CAD build for the part. Positions are in the model's coordinates, mm. Give positions to 0.01 mm unless a question says otherwise; leave off trailing zeros. Write each loop counter-clockwise with the first axis right and the second up, starting at its lowest first coordinate (ties: lowest second). Pieces come first, ordered by that corner, then holes. Notation, with made-up numbers: (60, -35) - (87, -35) arc R22 ccw to (87, -26) - close; hole circle Ø3 at (71, -11.5). An arc over 180 degrees is marked (long way). Answer as a JSON object with one key per item and string values.
from build123d import *

# Parameters (mm, degrees)
F0_R     = 10
F0_R_2   = 5
F1_DEPTH = 5
F3_DEPTH = 15
F4_R     = 5
F5_DEPTH = 24.90763


with BuildPart() as f1:
    # F0 (on Front) → F1 (new body)
    with BuildSketch(Plane.XZ):
        Circle(F0_R)
        Circle(F0_R_2, mode=Mode.SUBTRACT)
    extrude(amount=F1_DEPTH)

    # F2 (on Front) → F3 (join)
    with BuildSketch(Plane.XZ):
        with BuildLine():
            ThreePointArc((0, -10), (7.071068, -7.071068), (10, 0))
            ThreePointArc((10, 0), (7.071068, 7.071068), (0, 10))
            ThreePointArc((0, 10), (-10, 0), (0, -10))
        make_face()
        with BuildLine():
            ThreePointArc((0, 10), (7.071068, 7.071068), (10, 0))
            ThreePointArc((10, 0), (7.071068, -7.071068), (0, -10))
            Line((0, -10), (15, -10))
            Line((15, -10), (23.552744, -5))
            Line((23.552744, -5), (23.552744, 5))
            Line((23.552744, 5), (15, 10))
            Line((15, 10), (0, 10))
        make_face()
    extrude(amount=-F3_DEPTH)

    # F4 (on Front) → F5 (cut, symmetric)
    with BuildSketch(Plane.XZ):
        Circle(F4_R)
    extrude(amount=F5_DEPTH, both=True, mode=Mode.SUBTRACT)


solid = f1.part
(1) Saw through at B-B, the plane x = -4. Give the cut face in (y, z), and give its area (3 significant figures).
Answer key:
{"outline": "(-5, -9.17) - (15, -9.17) - (15, -3) - (-5, -3) - close; (-5, 3) - (15, 3) - (15, 9.17) - (-5, 9.17) - close", "area": "247 mm²"}
(2) Saw through at C-C, the plane y = 10.5. Give the cut face in (x, z).
Answer key:
{"outline": "(0, -10) - (15, -10) - (23.55, -5) - (23.55, 5) - (15, 10) - (0, 10) arc R10 ccw to start; hole circle Ø10 at (0, 0)"}
(3) Probe L1, parallel to Z at x = 0, y = -3.2; L2, parallel to Y at x = 16.5, z = 8; L3, parallel to X at y = 2.5, z = 1. List the from-to ranges inside material, lowest first. Write a range as [from, to].
Answer key:
{"L1": "z = [-10, -5], [5, 10]", "L2": "y = [0, 15]", "L3": "x = [-9.95, -4.9], [4.9, 23.55]"}
(4) Saw through at A-A, the plane z = -1.25. Give the cut face in (x, y), and give its area (3 significant figures).
Answer key:
{"outline": "(-9.92, -5) - (-4.84, -5) - (-4.84, 15) - (-9.92, 15) - close; (4.84, -5) - (9.92, -5) - (9.92, 0) - (23.55, 0) - (23.55, 15) - (4.84, 15) - close", "area": "408 mm²"}
(5) Flat gauge pins, fed straight in: P1, Ø1, axis at x = 17, z = 2, coming from the -Y side; P2, Ø4, axis at y = 5.5, z = 3.5, coming from the -X side; P3, Ø2, axis at y = 10, z = -7.5, coming from the -X side; P4, Ø8, axis at x = 0, z = 0, coming from the -Y side. Where does each tip first touch, or does it go through?
Answer key:
{"P1": "stops at y = 0", "P2": "stops at x = -9.89", "P3": "stops at x = -7.6", "P4": "passes through"}
(6) Saw through at D-D, the plane x = 12. Give the cut face in (y, z).
Answer key:
{"outline": "(0, -10) - (15, -10) - (15, 10) - (0, 10) - close"}
